from build123d import *

# Parameters (mm, degrees)
BOSS_EXTRUDE1_DEPTH = 30
SKETCH2_OUTSIDE_W   = 17.593
SKETCH2_OUTSIDE_H   = 38.81
CUT_EXTRUDE1_DEPTH  = 15
SKETCH3_OUTSIDE_W   = 22.31
SKETCH3_OUTSIDE_H   = 38.81
SKETCH3_OUTSIDE_R   = 2
CUT_EXTRUDE2_DEPTH  = 15


with BuildPart() as part:
    # Sketch1 → Boss-Extrude1 (new body)
    with BuildSketch(Plane(origin=(0, 0, 0), x_dir=(1, 0, 0), z_dir=(0, 1, 0))):
        with BuildLine():
            Line((-4.75, -0.283032593), (-4.75, 5.5))
            Line((-4.75, 5.5), (-6.75, 5.5))
            Line((-6.75, 5.5), (-6.75, 8.5))
            Line((-6.75, 8.5), (6.75, 8.5))
            Line((6.75, 8.5), (6.75, 5.5))
            Line((6.75, 5.5), (4.75, 5.5))
            Line((4.75, 5.5), (4.75, -0.283032593))
            ThreePointArc((4.75, -0.283032593), (0, 0), (-4.75, -0.283032593))
        make_face()
    extrude(amount=BOSS_EXTRUDE1_DEPTH)

    # Sketch2 outside → Cut-Extrude1 (cut)
    with BuildSketch(Plane(origin=(6.75, 0, 0), x_dir=(0, 0, -1), z_dir=(1, 0, 0))):
        with Locations((4.1085, 15)):
            Rectangle(SKETCH2_OUTSIDE_W, SKETCH2_OUTSIDE_H)
        Polygon((-0.283032593, 30), (8.5, 17.456529509), (8.5, 7.456529509), (-0.283032593, 0), align=None, mode=Mode.SUBTRACT)
    extrude(amount=-CUT_EXTRUDE1_DEPTH, mode=Mode.SUBTRACT)

    # Sketch3 outside → Cut-Extrude2 (cut)
    # profile 1 of 2: a face of its own
    with BuildSketch(Plane(origin=(0, 0, -8.5), x_dir=(-1, 0, 0), z_dir=(0, 0, -1))):
        with Locations((0, 15)):
            Rectangle(SKETCH3_OUTSIDE_W, SKETCH3_OUTSIDE_H)
        Polygon((-6.75, 17.456529509), (-0.894644938, 30), (0.894644938, 30), (6.75, 17.456529509), (6.75, 7.456529509), (0.894644938, 0), (-0.894644938, 0), (-6.75, 7.456529509), align=None, mode=Mode.SUBTRACT)
    # profile 2 of 2: a face of its own
    with BuildSketch(Plane(origin=(0, 0, -8.5), x_dir=(-1, 0, 0), z_dir=(0, 0, -1))):
        with Locations((0, 12.456529509)):
            Circle(SKETCH3_OUTSIDE_R)
    extrude(amount=-CUT_EXTRUDE2_DEPTH, mode=Mode.SUBTRACT)


solid = part.part
For this review, take the finished solid that the model builds, in its own axes (mm). A direction names the side the tool comes from. Coordinates: 2 decimals unless noted, no trailing zeros. Loops run counter-clockwise (first coordinate to the right, second up) from the corner with the lowest first, then second, coordinate; pieces in that order, holes last. Notation, with made-up numbers: (55, 82) - (77, 82) arc R27 cw to (77, 106) - close; hole circle Ø2 at (53.25, 55.25). An arc over 180 degrees is marked (long way). Use a Markdown table: item, result. Add a question column.
Item 1: Tool access review of faces 4 (the face through (3.346, 24.749, -2.006)), 5 (the face through (-4.75, 13, -3)), 6 (the face through (6, 13, -5.5)): name each direction out of +Z, -Z, +X, -X, +Y, -Y from which nothing blocks a thin tool from reaching the whole face with its end or side.
Item 2: For line 1 (X direction, y = 16.5, z = -0.5); line 2 (Z direction, x = -4.25, y = 11); line 3 (Z direction, x = 5.75, y = 14.25), list the stretches that pass through material, from the lowest coordinate up.
Item 3: We need section B-B (x = 0). Give the boundary of the cut face in (y, z), and give its area (3 significant figures).
Item 4: We need section C-C (z = -0.5). Give the boundary of the cut face in (x, y), and give its area (3 significant figures).
Item 5: Mouldability with a two-part tool opening along X and no side actions: class faces 1 (the face through (-6.18, 18.68, -6.35)), 2 (the face through (0.26, 14.44, -4.28)), 3 (the face through (0.09, 4.7, -5.25)) as pulls with the +X half, pulls with the -X half, needs draft (parallel to the pull), parting line crosses it, or undercut.
Item 6: Insertion check: pin 1 Ø1.5 at (x, z) = (5, -3.5) entering from -Y; pin 2 Ø4.5 at (y, z) = (11, -2.5) entering from +X; pin 3 Ø1 at (x, y) = (-5.5, 16.5) entering from +Z; pin 4 Ø3.5 at (x, y) = (0, 12.46) entering from -Z. Each pin has a flat end and moves straight along its axis. Give the tip position at first contact, or say it passes through.
Item 7: We need section A-A (y = 12.75). Give the boundary of the cut face in (x, z).
Item 8: We need section D-D (y = 9.75). Give the boundary of the cut face in (x, z).
Results list:
| question | item | result |
|---|---|---|
| 1 | face 4 | +Z, -Z, +X, +Y |
| 1 | face 5 | +Z, -X, +Y, -Y |
| 1 | face 6 | +Z, +X, +Y, -Y |
| 2 | line 1 | x = -4.75 to 4.75 |
| 2 | line 2 | z = -8.5 to 0.23 |
| 2 | line 3 | z = -8.5 to -5.5 |
| 3 | outline | (0.24, 0) - (7.46, -8.5) - (10.46, -8.5) - (10.46, 0) - close; (14.46, -8.5) - (17.46, -8.5) - (29.6, 0) - (14.46, 0) - close |
| 3 | area | 133 mm^2 |
| 4 | outline | (-4.75, 4.91) - (-1.42, 0.66) - (1.42, 0.66) - (4.75, 4.91) - (4.75, 21.74) - (1.42, 28.88) - (-1.42, 28.88) - (-4.75, 21.74) - close; hole circle Ø4 at (0, 12.46) |
| 4 | area | 218 mm^2 |
| 5 | face 1 | pulls with the -X half |
| 5 | face 2 | undercut |
| 5 | face 3 | needs draft |
| 6 | pin 1 | stops at y = 4.27 |
| 6 | pin 2 | stops at x = 4.75 |
| 6 | pin 3 | stops at z = -5.5 |
| 6 | pin 4 | passes through |
| 7 | outline | (-6.75, -8.5) - (-1.98, -8.5) - (-1.98, 0.05) arc R40 cw to (-4.75, 0.28) - (-4.75, -5.5) - (-6.75, -5.5) - close; (1.98, -8.5) - (6.75, -8.5) - (6.75, -5.5) - (4.75, -5.5) - (4.75, 0.28) arc R40 cw to (1.98, 0.05) - close |
| 8 | outline | (-6.75, -8.5) - (6.75, -8.5) - (6.75, -5.5) - (4.75, -5.5) - (4.75, 0.28) arc R40 cw to (-4.75, 0.28) - (-4.75, -5.5) - (-6.75, -5.5) - close |
